Geometry check sheet. Reference: the model listing, model coordinates, mm. Face numbers are marked on the shaded views. A direction names the side the tool comes from. Round coordinates to 2 decimals unless told otherwise and drop trailing zeros. Write each loop counter-clockwise with the first axis right and the second up, starting at its lowest first coordinate (ties: lowest second). Pieces come first, ordered by that corner, then holes. Notation, with made-up numbers: M -39.75,37 L 19.25,37 A14 cw 19.25,61 Z; hole C 50.25,6.5 d9. An arc over 180 degrees is marked long. Put each result on its own line as item: value. Start each with the question number.
(1) Tool access check on the marked faces 1 and 2. Record the directions out of +Z, -Z, +X, -X, +Y, -Y that give a thin tool (end or side, any length) a straight path to the whole face; none if there is none.
(2) Section check A-A on x = 33. Record the cut outline in (y, z).
(3) Gauge pin test, flat ends, axial feed: pin 1 (1.5 mm diameter, centred on x = 38.5, z = 4, fed in from -Y); pin 2 (4 mm diameter, centred on x = 30, z = -6.5, fed in from -Y); pin 3 (1.5 mm diameter, centred on x = 13, y = 1.5, fed in from -Z). Record the tip position at first contact, or that the pin passes through.
(4) Material ranges on probe 1 along X at (y, z) = (4.25, 4); probe 2 along Y at (x, z) = (15.5, 2.5); probe 3 along Y at (x, z) = (37.5, 8.75), recorded low to high.
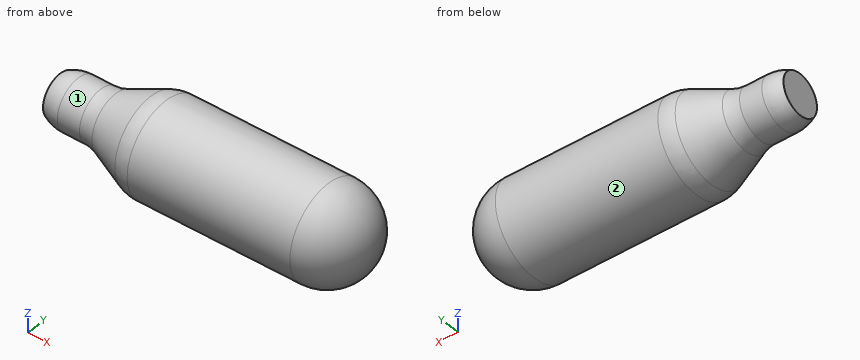
from build123d import *

# Parameters (mm, degrees)
F2_R = 9.5
F3_R = 7.62


with BuildPart() as f1:
    # F0 (on Front) → F1 (revolve)
    with BuildSketch(Plane.XZ):
        Polygon((0, 4.25), (0, 0), (64, 0), (64, 9.5), (19.793399, 9.5), (9.774541, 5.186723), (1.774541, 5.186723), align=None)
    revolve(axis=Axis((32, 0, 0), (1, 0, 0)))

    # F2
    f2_edges = [f1.edges().sort_by_distance(p)[0] for p in [
        (64, 0, -9.5),
    ]]
    fillet(f2_edges, radius=F2_R)

    # F3
    f3_edges = [f1.edges().sort_by_distance(p)[0] for p in [
        (19.793399, 0, -9.5),
        (1.774541, 0, -5.186723),
        (9.774541, 0, -5.186723),
    ]]
    fillet(f3_edges, radius=F3_R)


solid = f1.part
Answers follow:
1. face 1: -X
1. face 2: +X, -X
2. outline: C 0,0 d19
3. pin 1: stops at y = -8.93
3. pin 2: stops at y = -8.37
3. pin 3: stops at z = -6.77
4. probe 1: x = 11.28 to 62
4. probe 2: y = -7.23 to 7.23
4. probe 3: y = -3.7 to 3.7
